Geometry check sheet. Reference: the model listing, model coordinates, mm. Face numbers are marked on the shaded views. A direction names the side the tool comes from. Round coordinates to 2 decimals unless told otherwise and drop trailing zeros. Order: outer loops, then holes, each group sorted by start corner. A loop starts at its lowest first (then second) coordinate and runs counter-clockwise, first axis right, second up. Notation, with made-up numbers: (5.25, 66) - (40.25, 66) arc R16 cw to (40.25, 94) - close; hole circle Ø2 at (51, -11.5). An arc over 180 degrees is marked (long way). Return JSON: item names as keys, results as strings. Group by question number.
Q1. Sectioned sample at A-A, the plane x = -10. Record the cut outline in (y, z), then the cut area to 3 significant figures.
Q2. Material ranges on line 1 along X through (y, z) = (53.65, -60); line 2 along Z through (x, y) = (55, 53.75); line 3 along Z through (x, y) = (-10, -2.75), recorded low to high.
Q3. Sectioned sample at C-C, the plane x = -35. Record the cut outline in (y, z).
Q4. Tool access check on the marked faces 1, 2 and 3. Record the directions out of +Z, -Z, +X, -X, +Y, -Y that give a thin tool (end or side, any length) a straight path to the whole face; none if there is none.
Q5. Sectioned sample at B-B, the plane z = -115. Record the cut outline in (x, y).
Q6. Gauge pin test, flat ends, axial feed: pin 1 Ø5 at (y, z) = (-7, -4) entering from -X; pin 2 Ø4 at (x, z) = (9.5, -22.5) entering from +Y; pin 3 Ø7 at (x, z) = (90, -55) entering from +Y; pin 4 Ø7 at (x, z) = (90, -40) entering from -Y. Record the tip position at first contact, or that the pin passes through.
Q7. Sectioned sample at D-D, the plane z = 5. Record the cut outline in (x, y).
```python
from build123d import *

# Parameters (mm, degrees)
BOSS_EXTRUDE1_DEPTH   = 10
SKETCH2_W             = 20
SKETCH2_H             = 10
BOSS_EXTRUDE2_DEPTH   = 25
F_6_CLEARANCE_HOLE1_D = 4.3053
SKETCH5_W             = 135
SKETCH5_H             = 85
BOSS_EXTRUDE3_DEPTH   = 5
F_6_CLEARANCE_HOLE2_D = 4.3053
F_6_CLEARANCE_HOLE3_D = 4.3053


with BuildPart() as part:
    # Sketch1 → Boss-Extrude1 (new body)
    with BuildSketch(Plane(origin=(0, 0, 0), x_dir=(0, 0, -1), z_dir=(1, 0, 0))):
        with BuildLine():
            Line((-10, 0), (-10, -10))
            Line((-10, -10), (10, -10))
            Line((10, -10), (10, 0))
            ThreePointArc((10, 0), (13.886241397, 10.127382743), (23.549723757, 15.055248619))
            ThreePointArc((23.549723757, 15.055248619), (45.979641528, 26.493322625), (55, 50))
            Line((55, 50), (35, 50))
            ThreePointArc((35, 50), (31.113758603, 39.872617257), (21.450276243, 34.944751381))
            ThreePointArc((21.450276243, 34.944751381), (-0.979641528, 23.506677375), (-10, 0))
        make_face()
    extrude(amount=BOSS_EXTRUDE1_DEPTH)

    # Sketch2 → Boss-Extrude2 (add)
    with BuildSketch(Plane(origin=(10, 0, 0), x_dir=(0, 0, -1), z_dir=(1, 0, 0))):
        with Locations((0, -5)):
            Rectangle(SKETCH2_W, SKETCH2_H)
    extrude(amount=-BOSS_EXTRUDE2_DEPTH)

    # #6 Clearance Hole1 (through all)
    with Locations(Plane(origin=(0, 0, 0), x_dir=(1, 0, 0), z_dir=(0, 1, 0))):
        with Locations((-10, 5), (-10, -5)):
            Hole(F_6_CLEARANCE_HOLE1_D / 2)

    # Sketch5 → Boss-Extrude3 (add)
    with BuildSketch(Plane(origin=(0, 50, 0), x_dir=(1, 0, 0), z_dir=(0, 1, 0))):
        with Locations((27.5, 77.5)):
            Rectangle(SKETCH5_W, SKETCH5_H)
    extrude(amount=BOSS_EXTRUDE3_DEPTH)

    # #6 Clearance Hole2 (through all)
    with Locations(Plane(origin=(0, 55, 0), x_dir=(1, 0, 0), z_dir=(0, 1, 0))):
        with Locations((20, 115), (20, 60), (-35, 60), (-35, 115)):
            Hole(F_6_CLEARANCE_HOLE2_D / 2)

    # #6 Clearance Hole3 (through all)
    with Locations(Plane(origin=(0, 55, 0), x_dir=(1, 0, 0), z_dir=(0, 1, 0))):
        with Locations((90, 40), (55, 40), (55, 51.266063414), (90, 55)):
            Hole(F_6_CLEARANCE_HOLE3_D / 2)


solid = part.part
```
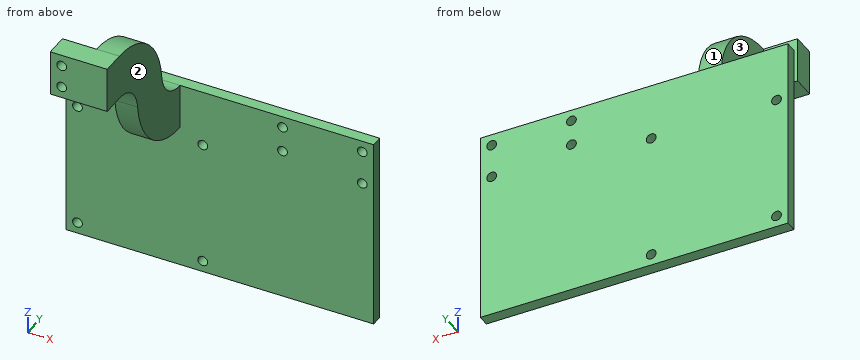
Reply:
{
 "1": {"outline": "(-10, -10) - (0, -10) - (0, -7.15) - (-10, -7.15) - close; (-10, -2.85) - (0, -2.85) - (0, 2.85) - (-10, 2.85) - close; (-10, 7.15) - (0, 7.15) - (0, 10) - (-10, 10) - close; (50, -120) - (55, -120) - (55, -35) - (50, -35) - close", "area": "539 mm^2"},
 "2": {"line 1": "-40 to -37.15, -32.85 to 17.85, 22.15 to 95", "line 2": "-120 to -53.42, -49.11 to -42.15, -37.85 to -35", "line 3": "-10 to -7.15, -2.85 to 2.85, 7.15 to 10"},
 "3": {"outline": "(50, -120) - (55, -120) - (55, -117.15) - (50, -117.15) - close; (50, -112.85) - (55, -112.85) - (55, -62.15) - (50, -62.15) - close; (50, -57.85) - (55, -57.85) - (55, -35) - (50, -35) - close"},
 "4": {"face 1": "+Z, +X, -X, +Y", "face 2": "+Z, -Z, +X, -Y", "face 3": "+Z, -Z, -X"},
 "5": {"outline": "(-40, 50) - (-37.15, 50) - (-37.15, 55) - (-40, 55) - close; (-32.85, 50) - (17.85, 50) - (17.85, 55) - (-32.85, 55) - close; (22.15, 50) - (95, 50) - (95, 55) - (22.15, 55) - close"},
 "6": {"pin 1": "x = -15", "pin 2": "y = 35.59", "pin 3": "y = 55", "pin 4": "y = 50"},
 "7": {"outline": "(-15, -10) - (-12.15, -10) - (-12.15, 0) - (-15, 0) - close; (-7.85, -10) - (10, -10) - (10, 18.07) - (0, 18.07) - (0, 0) - (-7.85, 0) - close"}
}
